from build123d import *

# Parameters (mm, degrees)
PAD002_DEPTH          = 40
SKETCH003_W           = 41
SKETCH003_H           = 41
SKETCH003_R           = 12.5
PAD001_DEPTH          = 33
SKETCH004_R           = 1.46
POCKET001_DEPTH       = 7
POCKET002_DEPTH       = 159.43263
POLARPATTERN_COUNT    = 4
SKETCH006_R           = 1.75
POCKET003_DEPTH       = 15
POLARPATTERN001_COUNT = 4


with BuildPart() as obj1:
    # Sketch007 → Pad002 (new body)
    with BuildSketch(Plane.XY):
        Polygon((-25, 12), (-25, -25), (12, -25), (12, 0), (0, 0), (0, 12), align=None)
    extrude(amount=PAD002_DEPTH)


with BuildPart() as cut:
    # Sketch003 → Pad001 (new body)
    with BuildSketch(Plane.XY):
        Rectangle(SKETCH003_W, SKETCH003_H)
        Circle(SKETCH003_R, mode=Mode.SUBTRACT)
    extrude(amount=PAD001_DEPTH)

    # Sketch004 → Pocket001 (cut)
    with BuildSketch(Plane.XY.offset(33)):
        with Locations((-15.5, 15.5)):
            Circle(SKETCH004_R)
        with Locations((15.5, 15.5)):
            Circle(SKETCH004_R)
        with Locations((15.5, -15.5)):
            Circle(SKETCH004_R)
        with Locations((-15.5, -15.5)):
            Circle(SKETCH004_R)
    extrude(amount=-POCKET001_DEPTH, mode=Mode.SUBTRACT)

    # Sketch005 → Pocket002 (cut, through all)
    with BuildSketch(Plane.XY.offset(26)):
        with BuildLine():
            ThreePointArc((-11, -15.5), (-12.318019, -12.318019), (-15.5, -11))
            Line((-15.5, -11), (-21.5, -11))
            Line((-21.5, -11), (-21.5, -21.5))
            Line((-21.5, -21.5), (-11, -21.5))
            Line((-11, -15.5), (-11, -21.5))
        make_face()
    pocket002 = extrude(amount=-POCKET002_DEPTH, mode=Mode.SUBTRACT)

    # PolarPattern: Pocket002 ×4 about axis
    polarpattern_axis = Axis((0, 0, 26), (0, 0, 1))
    for i in range(1, POLARPATTERN_COUNT):
        add(pocket002.rotate(polarpattern_axis, i * 360 / POLARPATTERN_COUNT), mode=Mode.SUBTRACT)

    # Sketch006 → Pocket003 (cut)
    with BuildSketch(Plane(origin=(0, 0, 0), x_dir=(1, 0, 0), z_dir=(0, 0, -1))):
        with Locations((-17, 0)):
            Circle(SKETCH006_R)
    pocket003 = extrude(amount=-POCKET003_DEPTH, mode=Mode.SUBTRACT)

    # PolarPattern001: Pocket003 ×4 about axis
    polarpattern001_axis = Axis((0, 0, 0), (0, 0, -1))
    for i in range(1, POLARPATTERN001_COUNT):
        add(pocket003.rotate(polarpattern001_axis, i * 360 / POLARPATTERN001_COUNT), mode=Mode.SUBTRACT)

    # Cut: cut obj1
    add(obj1.part, mode=Mode.SUBTRACT)


solid = cut.part
Check sheet for the modelled part. Datum: model origin and axes. Units: mm. A direction names the side the tool comes from. Coordinates: 2 decimals unless noted, no trailing zeros. Loops run counter-clockwise (first coordinate to the right, second up) from the corner with the lowest first, then second, coordinate; pieces in that order, holes last. Notation, with made-up numbers: (-19.5, 0) -> (15.5, 0) arc R28 ccw to (15.5, 33) -> close; hole circle Ø3 at (10, 32.5). An arc over 180 degrees is marked (long way). Answer in a Markdown table with one row per item.
1. Go/stop test with flat-tipped pins: pin 1 (4 mm diameter, centred on x = 15.5, y = -15.5, fed in from -Z); pin 2 (2.5 mm diameter, centred on x = 15.5, y = 15.5, fed in from -Z); pin 3 (13.5 mm diameter, centred on x = -15.5, z = 21.5, fed in from -Y); pin 4 (6 mm diameter, centred on y = 0.5, z = 25, fed in from -X). Record where each tip stops, or that it passes through.
Check values:
| item | result |
|---|---|
| pin 1 | stops at z = 26 |
| pin 2 | passes through |
| pin 3 | stops at y = 12 |
| pin 4 | stops at x = 12 |
2. Sectioned sample at B-B, the plane x = -16. Record the boundary of the cut face in (y, z), then the cut area to 3 significant figures.
Check values:
| item | result |
|---|---|
| outline | (12, 26) -> (14.13, 26) -> (14.13, 33) -> (12, 33) -> close; (16.87, 26) -> (20.5, 26) -> (20.5, 33) -> (16.87, 33) -> close |
| area | 40.3 mm2 |
3. Access from +Z, -Z, +X, -X, +Y, -Y to the whole of each face (thin tool, end or side, straight path). Record for faces 5 (the face through (-20.5, 16, 29)), 6 (the face through (1.06, 18.39, 7.4)), 7 (the face through (18, -11, 13)), 8 (the face through (17, 17, 26)), 9 (the face through (-15.7, 17.3, 26)).
Check values:
| item | result |
|---|---|
| face 5 | +Z, -Z, -X, +Y, -Y |
| face 6 | -Z |
| face 7 | -Z, +X, -Y |
| face 8 | -Z, +X, +Y |
| face 9 | -Z, -X, +Y |
4. Sectioned sample at D-D, the plane z = 8. Record the boundary of the cut face in (x, y), then the cut area to 3 significant figures.
Check values:
| item | result |
|---|---|
| outline | (-12.67, 12) -> (-3.5, 12) arc R12.5 cw to (12, -3.5) -> (12, -12.67) arc R4.5 cw to (15.5, -11) -> (20.5, -11) -> (20.5, 11) -> (15.5, 11) arc R4.5 cw to (11, 15.5) -> (11, 20.5) -> (-11, 20.5) -> (-11, 15.5) arc R4.5 cw to start; hole circle Ø3.5 at (0, 17); hole circle Ø3.5 at (17, 0) |
| area | 381 mm2 |
5. Material ranges on line 1 along Y through (x, z) = (15.5, 29.25); line 2 along Y through (x, z) = (17, 2), recorded low to high. Write a range as [from, to].
Check values:
| item | result |
|---|---|
| line 1 | y = [-20.5, -16.96], [-14.04, 14.04], [16.96, 20.5] |
| line 2 | y = [-11, -1.75], [1.75, 11] |
6. Sectioned sample at A-A, the plane y = -15.5. Record the boundary of the cut face in (x, z), then the cut area to 3 significant figures.
Check values:
| item | result |
|---|---|
| outline | (12, 26) -> (14.04, 26) -> (14.04, 33) -> (12, 33) -> close; (16.96, 26) -> (20.5, 26) -> (20.5, 33) -> (16.96, 33) -> close |
| area | 39.1 mm2 |
7. Release check for a two-part mould opening along Y. For faces 1 (the face through (18, 11, 13)), 2 (the face through (-11, 18, 13)), 3 (the face through (13.586, -11.427, 13.182)), 4 (the face through (16.893, 15.939, 29.549)) record: released by +Y, released by -Y, zero draft, split by the parting line, or undercut.
Check values:
| item | result |
|---|---|
| face 1 | released by +Y |
| face 2 | zero draft |
| face 3 | released by -Y |
| face 4 | undercut |
8. Sectioned sample at C-C, the plane z = 22.5. Record the boundary of the cut face in (x, y), then the cut area to 3 significant figures.
Check values:
| item | result |
|---|---|
| outline | (-12.67, 12) -> (-3.5, 12) arc R12.5 cw to (12, -3.5) -> (12, -12.67) arc R4.5 cw to (15.5, -11) -> (20.5, -11) -> (20.5, 11) -> (15.5, 11) arc R4.5 cw to (11, 15.5) -> (11, 20.5) -> (-11, 20.5) -> (-11, 15.5) arc R4.5 cw to start |
| area | 400 mm2 |
